The listing builds one solid part. Answer for the finished solid, in the listing's coordinates (mm). Face numbers are marked on the shaded views. A direction names the side the tool comes from. Round coordinates to 2 decimals unless told otherwise and drop trailing zeros. Loops run counter-clockwise (first coordinate to the right, second up) from the corner with the lowest first, then second, coordinate; pieces in that order, holes last. Notation, with made-up numbers: (9, 0) - (15, 0) arc R12 ccw to (15, 9) - close; hole circle Ø11 at (7.25, -22.5). An arc over 180 degrees is marked (long way). One line per item, written item: value.
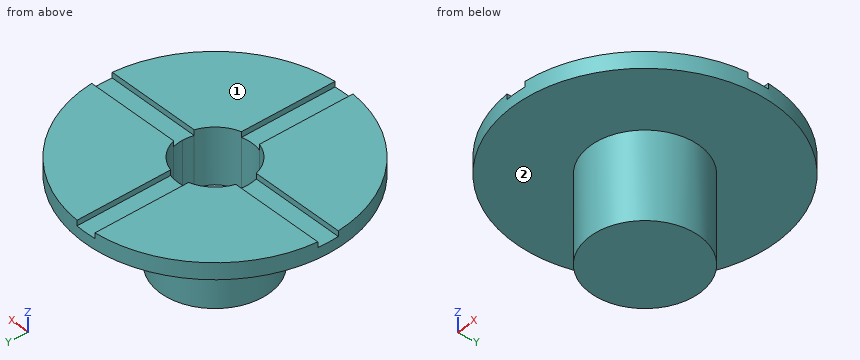
```python
from build123d import *

# Parameters (mm, degrees)
F0_R     = 12
F1_DEPTH = 1.5
F2_R     = 5
F3_DEPTH = 8
F5_DEPTH = 0.5
F6_DEPTH = 7
F7_R     = 2
F8_DEPTH = 3


with BuildPart() as f1:
    # F0 (on Top) → F1 (new body)
    with BuildSketch(Plane.XY):
        Circle(F0_R)
    extrude(amount=F1_DEPTH)

    # F2 (on face) → F3 (join)
    with BuildSketch(Plane(origin=(0, 0, 0), x_dir=(1, 0, 0), z_dir=(0, 0, -1))):
        Circle(F2_R)
    extrude(amount=F3_DEPTH)

    # F4 (on face) → F5 (cut)
    with BuildSketch(Plane.XY.offset(1.5)):
        with BuildLine():
            ThreePointArc((-0.95, 3.2802019755), (0, 3.415), (0.95, 3.2802019755))
            Line((0.95, 3.2802019755), (0.95, 11.9623367282))
            ThreePointArc((0.95, 11.9623367282), (0, 12), (-0.95, 11.9623367282))
            Line((-0.95, 11.9623367282), (-0.95, 3.2802019755))
        make_face()
        with BuildLine():
            ThreePointArc((-3.2802019755, -0.95), (-3.415, 0), (-3.2802019755, 0.95))
            Line((-3.2802019755, 0.95), (-11.9623367282, 0.95))
            ThreePointArc((-11.9623367282, 0.95), (-12, 0), (-11.9623367282, -0.95))
            Line((-11.9623367282, -0.95), (-3.2802019755, -0.95))
        make_face()
        with BuildLine():
            Line((0.95, -11.9623367282), (0.95, -3.2802019755))
            ThreePointArc((0.95, -3.2802019755), (0, -3.415), (-0.95, -3.2802019755))
            Line((-0.95, -3.2802019755), (-0.95, -11.9623367282))
            ThreePointArc((-0.95, -11.9623367282), (0, -12), (0.95, -11.9623367282))
        make_face()
        with BuildLine():
            ThreePointArc((3.2802019755, 0.95), (3.3811325578, 0.4797578836), (3.415, 0))
            ThreePointArc((3.415, 0), (3.3811325578, -0.4797578836), (3.2802019755, -0.95))
            Line((3.2802019755, -0.95), (11.9623367282, -0.95))
            ThreePointArc((11.9623367282, -0.95), (11.9905804851, -0.4753731487), (12, 0))
            ThreePointArc((12, 0), (11.9905804851, 0.4753731487), (11.9623367282, 0.95))
            Line((11.9623367282, 0.95), (3.2802019755, 0.95))
        make_face()
    extrude(amount=-F5_DEPTH, mode=Mode.SUBTRACT)

    # F4 (on face) → F6 (cut)
    with BuildSketch(Plane.XY.offset(1.5)):
        with BuildLine():
            ThreePointArc((3.2802019755, -0.95), (3.3811325578, -0.4797578836), (3.415, 0))
            ThreePointArc((3.415, 0), (3.3811325578, 0.4797578836), (3.2802019755, 0.95))
            ThreePointArc((3.2802019755, 0.95), (2.4147696578, 2.4147696578), (0.95, 3.2802019755))
            ThreePointArc((0.95, 3.2802019755), (0, 3.415), (-0.95, 3.2802019755))
            ThreePointArc((-0.95, 3.2802019755), (-2.4147696578, 2.4147696578), (-3.2802019755, 0.95))
            ThreePointArc((-3.2802019755, 0.95), (-3.415, 0), (-3.2802019755, -0.95))
            ThreePointArc((-3.2802019755, -0.95), (-2.4147696578, -2.4147696578), (-0.95, -3.2802019755))
            ThreePointArc((-0.95, -3.2802019755), (0, -3.415), (0.95, -3.2802019755))
            ThreePointArc((0.95, -3.2802019755), (2.4147696578, -2.4147696578), (3.2802019755, -0.95))
        make_face()
    extrude(amount=-F6_DEPTH, mode=Mode.SUBTRACT)

    # F7 (on face) → F8 (join)
    with BuildSketch(Plane.XY.offset(-5.5)):
        Circle(F7_R)
    extrude(amount=F8_DEPTH)


solid = f1.part
```
1) A cutting plane is placed at A-A on z = -3.5. Give the vertices of the cut face in (x, y) (3 decimals).
Final values:
outline: circle Ø10 at (0, 0); circle Ø4 at (0, 0); hole circle Ø6.83 at (0, 0)
2) A cutting plane is placed at B-B on x = 0. Give the vertices of the cut face in (y, z) (3 decimals).
Final values:
outline: (-12, 0) - (-5, 0) - (-5, -8) - (5, -8) - (5, 0) - (12, 0) - (12, 1) - (3.415, 1) - (3.415, -5.5) - (2, -5.5) - (2, -2.5) - (-2, -2.5) - (-2, -5.5) - (-3.415, -5.5) - (-3.415, 1) - (-12, 1) - close
3) A cutting plane is placed at C-C on z = -1. Give the vertices of the cut face in (x, y) (3 decimals), and give its area (3 significant figures).
Final values:
outline: circle Ø10 at (0, 0); hole circle Ø6.83 at (0, 0)
area: 41.9 mm2
4) For the marked faces 1 and 2, determine the directions among +Z, -Z, +X, -X, +Y, -Y from which every point of the face is accessible in a straight line to the end or side of a thin tool.
Final values:
face 1: +Z, +X, -X, +Y, -Y
face 2: -Z
5) A cutting plane is placed at D-D on y = 7.75. Give the vertices of the cut face in (x, z), and give its area (3 significant figures).
Final values:
outline: (-9.16, 0) - (9.16, 0) - (9.16, 1.5) - (0.95, 1.5) - (0.95, 1) - (-0.95, 1) - (-0.95, 1.5) - (-9.16, 1.5) - close
area: 26.5 mm2
6) Consider L1, parallel to X at y = -1.25, z = -5; L2, parallel to Z at x = 6, y = 4.5; L3, parallel to Y at x = -0.25, z = -1. Determine where each line is inside the solid, lowest interval first.
Final values:
L1: -4.84 to -3.18, -1.56 to 1.56, 3.18 to 4.84
L2: 0 to 1.5
L3: -4.99 to -3.41, 3.41 to 4.99
7) Each of these flat-tipped pins is pushed along its axis until it touches: pin 1 Ø12 at (x, y) = (4, -4) entering from -Z; pin 2 Ø3 at (x, z) = (-1, -3.5) entering from -Y; pin 3 Ø1.5 at (x, y) = (-8, 0) entering from +Z; pin 4 Ø3.5 at (x, y) = (-0.5, 0.5) entering from +Z. Where does it stop, or does it pass through?
Final values:
pin 1: z = -8
pin 2: y = -5
pin 3: z = 1
pin 4: z = -2.5
